CAD build for the part. Positions are in the model's coordinates, mm. Give positions to 0.01 mm unless a question says otherwise; leave off trailing zeros. Order: outer loops, then holes, each group sorted by start corner. A loop starts at its lowest first (then second) coordinate and runs counter-clockwise, first axis right, second up. Notation, with made-up numbers: (9.25, -27) -> (19.25, -27) arc R13 cw to (19.25, -12) -> close; hole circle Ø2 at (8.5, -38). An arc over 180 degrees is marked (long way). Use one line per item in the form item = value. Start each with the question number.
1) Probe line 1 (X direction, y = 15, z = 6.25); line 2 (X direction, y = 149, z = 1.5). List the from-to ranges inside material, lowest first.
2) Cut at A-A, the plane x = 155. Give the cut face in (y, z).
3) Drop a flat-ended pin along its axis: P1, Ø9, axis at x = 155, y = 15, coming from the +Z side. Give the stop position or say it passes through.
4) Cut at C-C, the plane z = 2.25. Give the cut face in (x, y).
5) Mould opens along X. For faces 1 (the face through (86, 170, 5)), 2 (the face through (0, 86, 5)), 3 (the face through (170, 84, 5)), 4 (the face through (162.154, 157.253, 5.07)) say: pulls with the +X half, pulls with the -X half, needs draft (parallel to the pull), parting line crosses it, or undercut.
Autodesk Inventor part; units mm, degrees
ref_plane "YZ Plane" through (0, 0, 0) normal (1, 0, 0) x (0, 1, 0)
ref_plane "XZ Plane" through (0, 0, 0) normal (0, 1, 0) x (-1, 0, 0)
ref_plane "XY Plane" through (0, 0, 0) normal (0, 0, 1) x (1, 0, 0)
sketch "Sketch1" plane through (0, 0, 0) normal (0, 0, 1) x (1, 0, 0)
  line L0 (0, 0) -> (170, 0)
  line L1 (170, 0) -> (170, 170)
  line L2 (170, 170) -> (0, 170)
  line L3 (0, 170) -> (0, 0)
  dimension "d0" = 170
  dimension "d1" = 170
extrude "Extrusion1" add sketch "Sketch1" along normal blind 10
sketch "Sketch2" plane through (0, 0, 10) normal (0, 0, 1) x (1, 0, 0)
  line L0 (170, 170) -> (0, 170)
  line L1 (0, 170) -> (0, 155)
  line L2 (0, 170) -> (0, 0)
  line L3 (0, 0) -> (170, 0)
  line L4 (0, 0) -> (0, 15)
  line L5 (0, 15) -> (155, 15)
  line L6 (155, 15) -> (155, 155)
  line L7 (155, 155) -> (15, 155)
  line L8 (15, 155) -> (15, 15)
  line L9 (15, 155) -> (30, 155)
  circle A0 centre (15, 155) radius 7.5
  circle A1 centre (155, 155) radius 7.5
  circle A2 centre (155, 15) radius 7.5
  circle A3 centre (15, 15) radius 7.5
  dimension "d4" = 15
  dimension "d5" = 15
  dimension "d6" = 155
  dimension "d7" = 140
  dimension "d8" = 140
  dimension "d9" = 140
  dimension "d10" = 15
  dimension "d11" = 15
  dimension "d12" = 15
  dimension "d13" = 15
extrude "Extrusion2" cut sketch "Sketch2" against normal blind 10 contours L8 A3 L5 | L5 A3 | L5 A3 L8 | A2 L6 L5 | L5 L6 A2 | A0 L7 L8 | L8 L7 A0 | A1 L7 L6 | L6 L7 A1
properties part number "AF"
Result:
q1.line_1 = 0 to 7.5, 22.5 to 147.5, 162.5 to 170
q1.line_2 = 0 to 10.5, 19.5 to 150.5, 159.5 to 170
q2.outline = (0, 0) -> (7.5, 0) -> (7.5, 10) -> (0, 10) -> close; (22.5, 0) -> (147.5, 0) -> (147.5, 10) -> (22.5, 10) -> close; (162.5, 0) -> (170, 0) -> (170, 10) -> (162.5, 10) -> close
q3.P1 = through
q4.outline = (0, 0) -> (170, 0) -> (170, 170) -> (0, 170) -> close; hole circle Ø15 at (15, 15); hole circle Ø15 at (15, 155); hole circle Ø15 at (155, 15); hole circle Ø15 at (155, 155)
q5.face_1 = needs draft
q5.face_2 = pulls with the -X half
q5.face_3 = pulls with the +X half
q5.face_4 = undercut
